For this review, take the finished solid that the model builds, in its own axes (mm). A direction names the side the tool comes from. Coordinates: 2 decimals unless noted, no trailing zeros. Write each loop counter-clockwise with the first axis right and the second up, starting at its lowest first coordinate (ties: lowest second). Pieces come first, ordered by that corner, then holes. Notation, with made-up numbers: (1, -29) - (41, -29) arc R18 cw to (41, -8) - close; hole circle Ø3 at (32.25, 7). An arc over 180 degrees is marked (long way). Use one line per item in the form item = value. Start each with the question number.
1) Tool access review of faces 1 (the flat face through (19, -12.7, 8)), 2 (the flat face through (4, -19, 19.05)), 3 (the flat face through (10, 0, 10)): name each direction out of +Z, -Z, +X, -X, +Y, -Y from which nothing blocks a thin tool from reaching the whole face with its end or side.
2) We need section B-B (x = 16). Give the boundary of the cut face in (y, z), plus the area to 3 significant figures.
3) For L1, parallel to Z at x = 6.25, y = -27.5; L2, parallel to Z at x = 8, y = -14; L3, parallel to Y at x = 13.25, z = 9.5, list the stretches that pass through material, from the lowest coordinate up. Write a range as from..to.
4) We need section C-C (z = 8.5). Give the boundary of the cut face in (x, y), plus the area to 3 significant figures.
5) Insertion check: P1, Ø4, axis at x = 5.5, y = -5, coming from the +Z side (3 decimals); P2, Ø6, axis at x = 20, y = -12.5, coming from the +Z side; P3, Ø5, axis at x = 3, z = 20.5, coming from the -Y side. Each pin has a flat end and moves straight along its axis. Give the tip position at first contact, or say it passes through.
6) We need section A-A (y = -24.5). Give the boundary of the cut face in (x, z).
7) We need section D-D (z = 15.5). Give the boundary of the cut face in (x, y).
```python
from build123d import *

# Parameters (mm, degrees)
F0_W     = 25.4
F0_H     = 6.35
F1_DEPTH = 38.1
F3_DEPTH = 12.7
F5_DEPTH = 12.7


with BuildPart() as f1:
    # F0 (on Front) → F1 (new body)
    with BuildSketch(Plane.XZ):
        Polygon((0, 25.4), (0, 6.35), (25.4, 6.35), align=None)
        with Locations((12.7, 3.175)):
            Rectangle(F0_W, F0_H)
    extrude(amount=F1_DEPTH)

    # F2 (on face) → F3 (cut)
    with BuildSketch(Plane.XZ.offset(38.1)):
        Polygon((0, 25.4), (0, 6.35), (25.4, 6.35), align=None)
    extrude(amount=-F3_DEPTH, mode=Mode.SUBTRACT)

    # F4 (on face) → F5 (cut)
    with BuildSketch(Plane.XZ.offset(25.4)):
        Polygon((8.466667, 19.05), (0, 25.4), (0, 19.05), align=None)
        Polygon((25.4, 6.35), (16.933333, 12.7), (16.933333, 6.35), align=None)
    extrude(amount=-F5_DEPTH, mode=Mode.SUBTRACT)


solid = f1.part
```
Determined:
q1.face_1 = +Z, +X, -Y
q1.face_2 = +Z, +X, -X, -Y
q1.face_3 = +Z, -Z, +X, -X, +Y
q2.outline = (-38.1, 0) - (0, 0) - (0, 13.4) - (-25.4, 13.4) - (-25.4, 6.35) - (-38.1, 6.35) - close
q2.area = 421 mm²
q3.L1 = 0..6.35
q3.L2 = 0..19.05
q3.L3 = -25.4..0
q4.outline = (0, -25.4) - (16.93, -25.4) - (16.93, -12.7) - (22.53, -12.7) - (22.53, 0) - (0, 0) - close
q4.area = 501 mm²
q5.P1 = 22.775
q5.P2 = 12.65
q5.P3 = -25.4
q6.outline = (0, 0) - (25.4, 0) - (25.4, 6.35) - (16.93, 6.35) - (16.93, 12.7) - (8.47, 19.05) - (0, 19.05) - close
q7.outline = (0, -25.4) - (13.2, -25.4) - (13.2, 0) - (0, 0) - close
